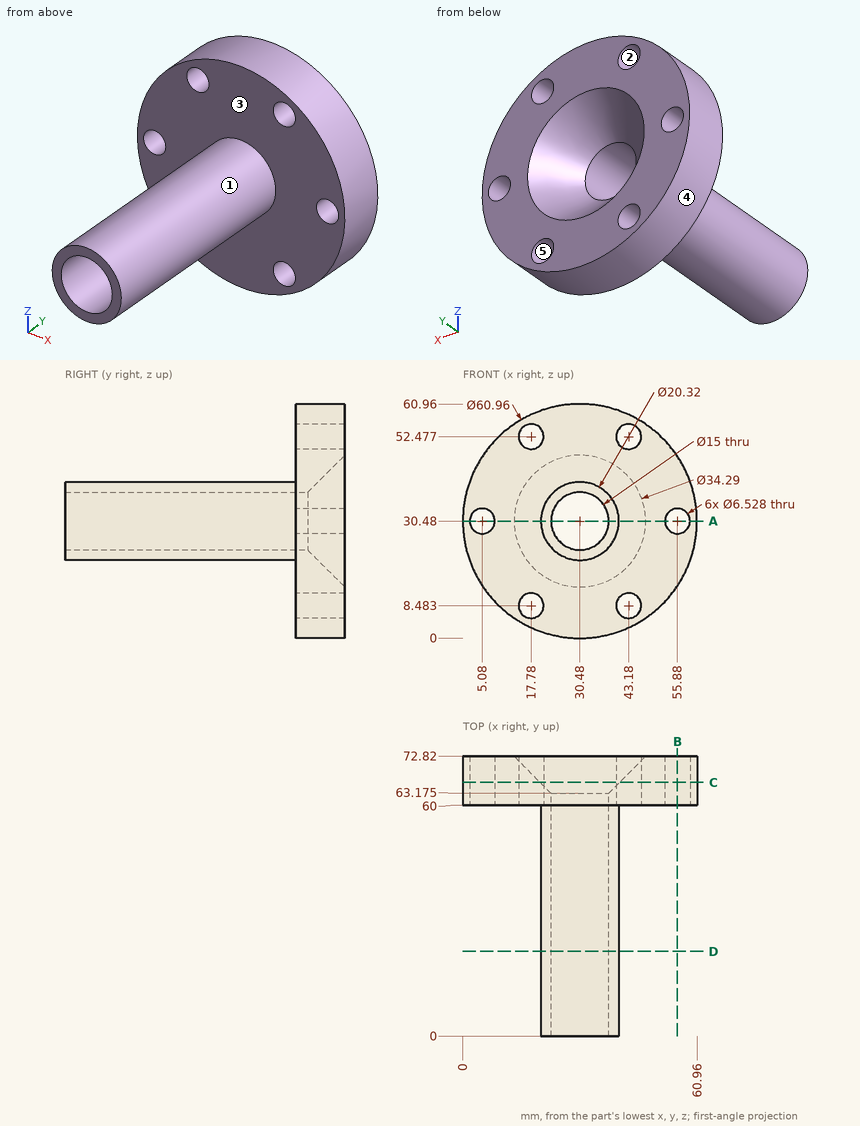
Can you work these out from the drawing? Everything is in mm from the part's minimum corner. A direction names the side the tool comes from. Give positions to 0.01 mm unless a question says otherwise; leave off trailing zeros. Loops run counter-clockwise (first coordinate to the right, second up) from the corner with the lowest first, then second, coordinate; pieces in that order, holes last. Notation, with made-up numbers: (26.5, -7.5) - (77.5, -7.5) arc R22 cw to (77.5, 15.5) - close; hole circle Ø7 at (-23.5, -31). An arc over 180 degrees is marked (long way). Answer as a JSON object with one key per item and string values.
Q1. Will these pins go through, and if not, where does the flat tip stop? P1, Ø12, axis at x = 27, y = 61, coming from the -Z side; P2, Ø1, axis at y = 62, z = 32.5, coming from the -X side; P3, Ø10.5, axis at x = 43.18, z = 8.48, coming from the -Y side; P4, Ø1.5, axis at x = 37, y = 61, coming from the -Z side.
Geometry says:
{"P1": "z = 0", "P2": "x = 0.04", "P3": "y = 60", "P4": "z = 0.55"}
Q2. Imagine slicing it at C-C on y = 66. Give the number of separate pieces and of enclosed holes in the cut face, plus the area to 3 significant figures.
Geometry says:
{"separate pieces": "1", "enclosed holes": "7", "area": "2,380 mm²"}
Q3. Imagine slicing it at D-D on y = 22. Write out the boundary of the cut face in (x, z).
Geometry says:
{"outline": "circle Ø20.32 at (30.48, 30.48); hole circle Ø15 at (30.48, 30.48)"}
Q4. Which directions (+Z, -Z, +X, -X, +Y, -Y) give clear straight access to the entire face, cutting with the end or side of a thin tool? Please do the marked faces 1 and 2.
Geometry says:
{"face 1": "-Y", "face 2": "+Y, -Y"}
Q5. If I drill on L1, parallel to Y at x = 5.5, z = 40.5; L2, parallel to Z at x = 17.78, y = 67.25; L3, parallel to Z at x = 30.48, y = 40, over which ranges is the centre line in solid material (lowest first)?
Geometry says:
{"L1": "60 to 72.82", "L2": "2.77 to 5.22, 11.75 to 49.21, 55.74 to 58.19", "L3": "20.32 to 22.98, 37.98 to 40.64"}
Q6. Imagine slicing it at A-A on z = 30.48. Write out the boundary of the cut face in (x, y) (1 decimal), plus the area to 3 significant figures.
Geometry says:
{"outline": "(0, 60) - (1.8, 60) - (1.8, 72.8) - (0, 72.8) - close; (8.3, 60) - (20.3, 60) - (20.3, 0) - (23, 0) - (23, 63.2) - (13.3, 72.8) - (8.3, 72.8) - close; (38, 0) - (40.6, 0) - (40.6, 60) - (52.6, 60) - (52.6, 72.8) - (47.6, 72.8) - (38, 63.2) - close; (59.1, 60) - (61, 60) - (61, 72.8) - (59.1, 72.8) - close", "area": "648 mm²"}
Q7. Imagine slicing it at B-B on x = 55.88. Write out the boundary of the cut face in (y, z), plus the area to 3 significant figures.
Geometry says:
{"outline": "(60, 13.63) - (72.82, 13.63) - (72.82, 27.22) - (60, 27.22) - close; (60, 33.74) - (72.82, 33.74) - (72.82, 47.33) - (60, 47.33) - close", "area": "348 mm²"}
Q8. If we mould it in two halves opening along X, with no side actions, what happens to the marked faces 3, 4 and 5? For each: pulls with the +X half, pulls with the -X half, needs draft (parallel to the pull), parting line crosses it, or undercut.
Geometry says:
{"face 3": "needs draft", "face 4": "parting line crosses it", "face 5": "undercut"}
